from build123d import *

# Parameters (mm, degrees)
SKETCH1_R           = 25
BOSS_EXTRUDE1_DEPTH = 60
CUT_EXTRUDE1_DEPTH  = 74
SKETCH3_R           = 20
BOSS_EXTRUDE2_DEPTH = 120


with BuildPart() as part:
    # Sketch1 → Boss-Extrude1 (new body)
    with BuildSketch(Plane.XY):
        with BuildLine():
            Line((64.94754869, 34.367143049), (196.507423933, 35.326035965))
            Line((196.507423933, 35.326035965), (196.511673709, -34.673963906))
            Line((196.511673709, -34.673963906), (63.689894991, -34.673963906))
            ThreePointArc((63.689894991, -34.673963906), (42.633771657, -37.171737248), (22.746391068, -44.526415681))
            ThreePointArc((22.746391068, -44.526415681), (-49.999854067, 0.120802809), (22.961281527, 44.415983054))
            ThreePointArc((22.961281527, 44.415983054), (43.342950879, 36.836730802), (64.94754869, 34.367143049))
        make_face()
        with Locations(Location((0, 0, 0), (0, 0, 180))):
            Circle(SKETCH1_R, mode=Mode.SUBTRACT)
    extrude(amount=BOSS_EXTRUDE1_DEPTH)

    # Sketch2 → Cut-Extrude1 (cut)
    with BuildSketch(Plane(origin=(196.509567891, 0.011930308, 0), x_dir=(0, 0, -1), z_dir=(0.9999999981570824, 6.0711079910172726e-05, 0))):
        Polygon((-60, 15.314105722), (-40.419671978, 35.314105722), (-60, 35.314105722), align=None)
        Polygon((0, 35.314105722), (-21.759605821, 35.314105722), (0, 17.974594403), align=None)
        Polygon((-40.419671978, -34.685894278), (-60, -12.535294787), (-60, -34.685894278), align=None)
        Polygon((0, -34.685894278), (0, -16.195205155), (-18.490689122, -34.685894278), align=None)
    extrude(amount=-CUT_EXTRUDE1_DEPTH, mode=Mode.SUBTRACT)

    # Sketch3 → Boss-Extrude2 (add)
    with BuildSketch(Plane(origin=(196.509567891, 0.011930308, 0), x_dir=(0, 0, -1), z_dir=(0.9999999981570824, 6.0711079910172726e-05, 0))):
        with Locations(Location((-31.0896389, 0, 0), (0, 0, 90))):
            Circle(SKETCH3_R)
    extrude(amount=BOSS_EXTRUDE2_DEPTH)


solid = part.part
CAD build for the part. Positions are in the model's coordinates, mm. A direction names the side the tool comes from. Coordinates: 2 decimals unless noted, no trailing zeros. Order: outer loops, then holes, each group sorted by start corner. A loop starts at its lowest first (then second) coordinate and runs counter-clockwise, first axis right, second up.
Item 1: Pin check, flat tips, straight feed: pin 1 Ø15.5 at (y, z) = (-22, 53) entering from +X; pin 2 Ø12 at (x, y) = (247.5, 28) entering from +Z; pin 3 Ø3 at (y, z) = (-3.5, 22.5) entering from -X; pin 4 Ø8 at (x, z) = (249.5, 11) entering from -Y. Stop position of each tip, or through.
Check sheet entries:
pin 1: stops at x = 196.51
pin 2: passes through
pin 3: stops at x = -49.96
pin 4: stops at y = -11.86
Item 2: Band-saw the part on D-D on z = 5. List the corners of the cut face in (x, y).
Check sheet entries:
outline: (22.75, -44.53) arc R90 cw to (63.69, -34.67) - (122.51, -34.67) - (122.51, -21.19) - (196.51, -21.18) - (196.51, 21.97) - (122.51, 21.97) - (122.51, 34.79) - (64.95, 34.37) arc R90 cw to (22.96, 44.42) arc R50 ccw (long way) to start; hole circle Ø50 at (0, 0)
Item 3: Two-plate mould, pull along X, no slides. Class faces 3 (the face through (42.923, -37.103, 29.58)), 4 (the face through (255.67, 19.09, 37.1)), 5 (the face through (-23.846, -7.509, 29.58)), 6 (the face through (-49.983, -1.311, 29.58)): +X half, -X half, draft (parallel to the pull), parting line (faces both ways), or undercut.
Check sheet entries:
face 3: +X half
face 4: draft
face 5: undercut
face 6: parting line
Item 4: 3-axis set-ups, long thin cutter, end or side, ignore diameter. For faces 1 (the face through (116, -34.674, 30)), 2 (the face through (48, 1, 60)): which of +Z, -Z, +X, -X, +Y, -Y reach the whole face in a straight line?
Check sheet entries:
face 1: +Z, -Z, +X, -Y
face 2: +Z, +X, -X, +Y, -Y
Item 5: Band-saw the part on B-B on z = 48. List the corners of the cut face in (x, y), plus the area to 3 significant figures.
Check sheet entries:
outline: (22.75, -44.53) arc R90 cw to (63.69, -34.67) - (122.51, -34.67) - (122.51, -26.1) - (196.51, -26.1) - (196.51, -10.67) - (316.51, -10.66) - (316.51, 10.7) - (196.51, 10.69) - (196.51, 27.58) - (122.51, 27.58) - (122.51, 34.79) - (64.95, 34.37) arc R90 cw to (22.96, 44.42) arc R50 ccw (long way) to start; hole circle Ø50 at (0, 0)
area: 17,900 mm2
Item 6: Drill centre lines: L1, parallel to X at y = 1, z = 37.5; L2, parallel to Y at x = 0, z = 46; L3, parallel to X at y = -13, z = 46.5. Where is each one in solid material? Low to high.
Check sheet entries:
L1: x = -49.99 to -24.98, 24.98 to 316.51
L2: y = -50 to -25, 25 to 50
L3: x = -48.28 to -21.35, 21.35 to 196.51
Item 7: Band-saw the part on A-A on x = 0. List the corners of the cut face in (y, z), plus the area to 3 significant figures.
Check sheet entries:
outline: (-50, 0) - (-25, 0) - (-25, 60) - (-50, 60) - close; (25, 0) - (50, 0) - (50, 60) - (25, 60) - close
area: 3,000 mm2
Item 8: Band-saw the part on C-C on x = 186.5. List the corners of the cut face in (y, z), plus the area to 3 significant figures.
Check sheet entries:
outline: (-34.67, 18.49) - (-16.18, 0) - (17.99, 0) - (35.25, 21.67) - (35.25, 40.49) - (15.33, 60) - (-12.52, 60) - (-34.67, 40.42) - close
area: 3,430 mm2
